Geometry: final body of the model. Coordinates: model frame, mm. Round coordinates to 2 decimals unless told otherwise and drop trailing zeros. Write each loop counter-clockwise with the first axis right and the second up, starting at its lowest first coordinate (ties: lowest second). Pieces come first, ordered by that corner, then holes. Notation, with made-up numbers: (-40, -18.5) -> (5, -18.5) arc R31 cw to (5, 19.5) -> close; hole circle Ø2 at (52, 88). An arc over 180 degrees is marked (long way). Use one line per item in the form item = value. Start each with the question number.
1. Pin query (flat end, axial travel): pin 1 Ø2 at (x, y) = (281.5, 8) entering from -Z; pin 2 Ø2 at (x, z) = (67.5, 15.5) entering from -Y; pin 3 Ø10 at (x, y) = (467.5, 28.5) entering from -Z. Return the tip coordinate at first contact, or that it passes through.
2. Cut plane B-B, the plane z = -9.5. Return the cut outline in (x, y), plus the area to 3 significant figures.
3. Line query: L1, parallel to Y at x = 296, z = -15.5; L2, parallel to Z at x = 364, y = 25; L3, parallel to Y at x = 456, z = 9. Output: solid intervals per line, ascending.
4. Cut plane C-C, the plane y = 27. Return the cut outline in (x, z).
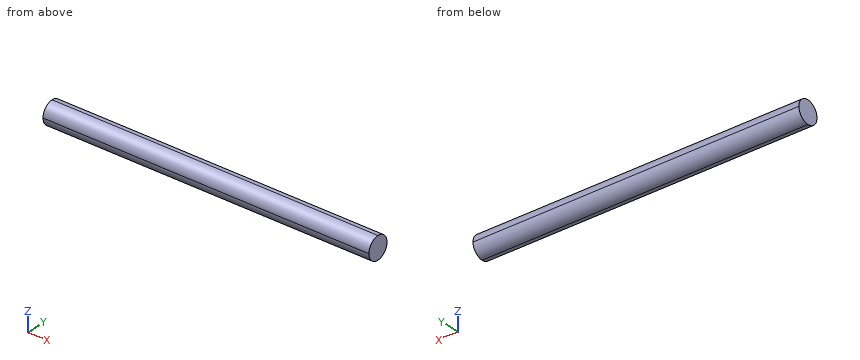
Autodesk Inventor part; units mm, degrees
ref_plane "YZ Plane" through (0, 0, 0) normal (1, 0, 0) x (0, 1, 0)
sketch "1.90 Caprail" plane through (0, 0, 0) normal (0, 0, 1) x (1, 0, 0)
  line L0 (-57.7384, 25.6152) -> (-57.7384, 36.7912) construction
  arc A0 (-65.9934, 36.7912) -> (-67.5174, 35.2672) centre (-65.9934, 35.2672) ccw
  arc A1 (-47.9594, 35.2672) -> (-49.4834, 36.7912) centre (-49.4834, 35.2672) ccw
  arc A2 (-69.8345, 6.4876) -> (-69.016, 6.9384) centre (-69.5494, 6.9384) ccw
  line L1 (-69.016, 6.9384) -> (-69.016, 35.2672)
  arc A3 (-65.9934, 38.2898) -> (-69.016, 35.2672) centre (-65.9934, 35.2672) ccw
  line L2 (-65.9934, 38.2898) -> (-49.4834, 38.2898)
  arc A4 (-46.4608, 35.2672) -> (-49.4834, 38.2898) centre (-49.4834, 35.2672) ccw
  line L3 (-46.4608, 35.2672) -> (-46.4608, 6.9384)
  arc A5 (-46.4608, 6.9384) -> (-45.6423, 6.4876) centre (-45.9274, 6.9384) ccw
  arc A6 (-45.6423, 6.4876) -> (-69.8345, 6.4876) centre (-57.7384, 25.6152) ccw
  line L4 (-47.9594, 6.9384) -> (-47.9594, 35.2672)
  line L5 (-49.4834, 36.7912) -> (-65.9934, 36.7912)
  line L6 (-67.5174, 35.2672) -> (-67.5174, 6.9384)
  arc A7 (-70.5058, 5.1455) -> (-67.5174, 6.9384) centre (-69.5494, 6.9384) ccw
  arc A8 (-47.9594, 6.9384) -> (-44.9711, 5.1455) centre (-45.9274, 6.9384) ccw
  arc A9 (-70.5083, 5.1411) -> (-44.9685, 5.1411) centre (-57.7384, 25.6152) ccw
  circle A10 centre (-57.7384, 25.6152) radius 24.13 construction
  arc A11 (-70.5058, 5.1455) -> (-70.5083, 5.1411) centre (-70.507, 5.1433) ccw
  arc A12 (-44.9685, 5.1411) -> (-44.9711, 5.1455) centre (-44.9699, 5.1433) ccw
  point P0 (-47.9594, 36.7912)
  point P1 (-67.5174, 36.7912)
  dimension "d0" = 48.26
  dimension "d1" = 19.558
  dimension "d2" = 2.032
  dimension "d3" = 11.176
  dimension "d4" = 1.524
  dimension "d5" = 1.4986
  dimension "d6" = 0.0025
sketch "1.66 Caprail" plane through (0, 0, 0) normal (0, 0, 1) x (1, 0, 0)
  arc A0 (55.7245, -3.4499) -> (81.6283, -3.4499) centre (68.6764, 13.1843) ccw
  arc A1 (55.7275, -3.4458) -> (58.8974, -1.7623) centre (56.8654, -1.7623) ccw
  arc A2 (78.4554, -1.7623) -> (81.6253, -3.4458) centre (80.4874, -1.7623) ccw
  line L0 (58.8974, -1.7623) -> (58.8974, 20.8043)
  line L1 (60.4214, 22.3283) -> (76.9314, 22.3283)
  line L2 (78.4554, 20.8043) -> (78.4554, -1.7623)
  line L3 (68.6764, 22.3283) -> (68.6764, 13.1843) construction
  arc A3 (60.4214, 22.3283) -> (58.8974, 20.8043) centre (60.4214, 20.8043) ccw
  arc A4 (78.4554, 20.8043) -> (76.9314, 22.3283) centre (76.9314, 20.8043) ccw
  arc A5 (79.954, -1.7623) -> (80.8181, -2.1808) centre (80.4874, -1.7623) ccw
  line L4 (79.954, -1.7623) -> (79.954, 20.8043)
  arc A6 (79.954, 20.8043) -> (76.9314, 23.8269) centre (76.9314, 20.8043) ccw
  line L5 (76.9314, 23.8269) -> (60.4214, 23.8269)
  arc A7 (60.4214, 23.8269) -> (57.3988, 20.8043) centre (60.4214, 20.8043) ccw
  line L6 (57.3988, 20.8043) -> (57.3988, -1.7623)
  arc A8 (56.5347, -2.1808) -> (57.3988, -1.7623) centre (56.8654, -1.7623) ccw
  arc A9 (80.8181, -2.1808) -> (56.5347, -2.1808) centre (68.6764, 13.1843) ccw
  circle A10 centre (68.6764, 13.1843) radius 21.082 construction
  arc A11 (55.7275, -3.4458) -> (55.7245, -3.4499) centre (55.7261, -3.4479) ccw
  arc A12 (81.6283, -3.4499) -> (81.6253, -3.4458) centre (81.6268, -3.4479) ccw
  point P0 (58.8974, 22.3283)
  point P1 (78.4554, 22.3283)
  dimension "d7" = 42.164
  dimension "d8" = 19.558
  dimension "d9" = 9.144
  dimension "d10" = 2.032
  dimension "d11" = 1.524
  dimension "d12" = 1.4986
  dimension "d13" = 0.0025
sketch "1.50 Caprail" plane through (0, 0, 0) normal (0, 0, 1) x (1, 0, 0)
  arc A0 (154.6368, -0.6357) -> (180.8596, -0.6357) centre (167.7482, 13.1843) ccw
  arc A1 (154.6402, -0.6319) -> (157.9692, 0.9323) centre (155.9372, 0.9323) ccw
  arc A2 (177.5272, 0.9323) -> (180.8562, -0.6319) centre (179.5592, 0.9323) ccw
  circle A3 centre (167.7482, 13.1843) radius 19.05 construction
  arc A4 (179.0258, 0.9323) -> (179.9294, 0.5483) centre (179.5592, 0.9323) ccw
  line L0 (179.0258, 0.9323) -> (179.0258, 23.0903)
  arc A5 (179.0258, 23.0903) -> (176.0032, 26.1129) centre (176.0032, 23.0903) ccw
  line L1 (176.0032, 26.1129) -> (159.4932, 26.1129)
  arc A6 (159.4932, 26.1129) -> (156.4706, 23.0903) centre (159.4932, 23.0903) ccw
  line L2 (156.4706, 23.0903) -> (156.4706, 0.9323)
  arc A7 (155.567, 0.5483) -> (156.4706, 0.9323) centre (155.9372, 0.9323) ccw
  arc A8 (179.9294, 0.5483) -> (155.567, 0.5483) centre (167.7482, 13.1843) ccw
  line L3 (157.9692, 0.9323) -> (157.9692, 23.0903)
  line L4 (159.4932, 24.6143) -> (176.0032, 24.6143)
  line L5 (177.5272, 23.0903) -> (177.5272, 0.9323)
  arc A9 (159.4932, 24.6143) -> (157.9692, 23.0903) centre (159.4932, 23.0903) ccw
  arc A10 (177.5272, 23.0903) -> (176.0032, 24.6143) centre (176.0032, 23.0903) ccw
  line L6 (167.7482, 24.6143) -> (167.7482, 13.1843) construction
  arc A11 (154.6402, -0.6319) -> (154.6368, -0.6357) centre (154.6385, -0.6339) ccw
  arc A12 (180.8596, -0.6357) -> (180.8562, -0.6319) centre (180.8578, -0.6339) ccw
  point P0 (157.9692, 24.6143)
  point P1 (177.5272, 24.6143)
  dimension "d14" = 38.1
  dimension "d15" = 19.558
  dimension "d16" = 2.032
  dimension "d17" = 1.524
  dimension "d18" = 11.43
  dimension "d19" = 1.4986
  dimension "d20" = 0.0025
sketch "1.90 Caprail Outside Edge" plane through (0, 0, 0) normal (0, 0, 1) x (1, 0, 0)
  arc A0 (8.6191, 38.6174) -> (-17.175, 38.6174) centre (-4.278, 59.0116) ccw
  line L0 (5.501, 40.3348) -> (5.501, 68.5975)
  line L1 (3.977, 70.1215) -> (-12.533, 70.1215)
  line L2 (-14.057, 68.5975) -> (-14.057, 40.3348)
  line L3 (-4.278, 59.0116) -> (-4.278, 70.1215) construction
  arc A1 (-17.175, 38.6174) -> (-14.057, 40.3348) centre (-16.089, 40.3348) ccw
  arc A2 (5.501, 40.3348) -> (8.6191, 38.6174) centre (7.533, 40.3348) ccw
  arc A3 (-12.533, 70.1215) -> (-14.057, 68.5975) centre (-12.533, 68.5975) ccw
  arc A4 (5.501, 68.5975) -> (3.977, 70.1215) centre (3.977, 68.5975) ccw
  point P0 (5.501, 70.1215)
  point P1 (-14.057, 70.1215)
  point P2 (-14.057, 36.9519)
  point P3 (5.501, 36.9519)
  dimension "d21" = 13.02
  dimension "d22" = 19.558
  dimension "d23" = 24.13
  dimension "d24" = 2.032
  dimension "d25" = 1.524
sketch "1.66 Caprail Outside Edge" plane through (0, 0, 0) normal (0, 0, 1) x (1, 0, 0)
  arc A0 (-64.2087, 6.8983) -> (-90.3503, 6.8983) centre (-77.2795, 23.4393) ccw
  line L0 (-67.5005, 8.4926) -> (-67.5005, 30.9932)
  line L1 (-69.0245, 32.5172) -> (-85.5345, 32.5172)
  line L2 (-87.0585, 30.9932) -> (-87.0585, 8.4926)
  line L3 (-77.2795, 23.4393) -> (-77.2795, 32.5172) construction
  arc A1 (-90.3503, 6.8983) -> (-87.0585, 8.4926) centre (-89.0905, 8.4926) ccw
  arc A2 (-67.5005, 8.4926) -> (-64.2087, 6.8983) centre (-65.4685, 8.4926) ccw
  arc A3 (-85.5345, 32.5172) -> (-87.0585, 30.9932) centre (-85.5345, 30.9932) ccw
  arc A4 (-67.5005, 30.9932) -> (-69.0245, 32.5172) centre (-69.0245, 30.9932) ccw
  point P0 (-67.5005, 32.5172)
  point P1 (-87.0585, 32.5172)
  point P2 (-87.0585, 4.7625)
  point P3 (-67.5005, 4.7625)
  dimension "d26" = 12.004
  dimension "d27" = 19.558
  dimension "d28" = 21.082
  dimension "d29" = 2.032
  dimension "d30" = 1.524
sketch "1.50 Caprail Outside Edge" plane through (0, 0, 0) normal (0, 0, 1) x (1, 0, 0)
  arc A0 (-129.2922, 11.7711) -> (-155.7348, 11.7711) centre (-142.5135, 25.486) ccw
  line L0 (-132.7345, 13.234) -> (-132.7345, 35.4784)
  line L1 (-134.2585, 37.0024) -> (-150.7685, 37.0024)
  line L2 (-152.2925, 35.4784) -> (-152.2925, 13.234)
  line L3 (-142.5135, 25.486) -> (-142.5135, 37.0024) construction
  arc A1 (-155.7348, 11.7711) -> (-152.2925, 13.234) centre (-154.3245, 13.234) ccw
  arc A2 (-132.7345, 13.234) -> (-129.2922, 11.7711) centre (-130.7025, 13.234) ccw
  arc A3 (-150.7685, 37.0024) -> (-152.2925, 35.4784) centre (-150.7685, 35.4784) ccw
  arc A4 (-132.7345, 35.4784) -> (-134.2585, 37.0024) centre (-134.2585, 35.4784) ccw
  point P0 (-132.7345, 37.0024)
  point P1 (-152.2925, 37.0024)
  point P2 (-152.2925, 9.1375)
  point P3 (-132.7345, 9.1375)
  dimension "d31" = 7.5336
  dimension "d32" = 19.558
  dimension "d33" = 19.05
  dimension "d34" = 2.032
  dimension "d35" = 1.524
sketch "Sketch1" plane through (0, 0, 0) normal (0, 0, 1) x (1, 0, 0)
  line L0 (0, 0) -> (609.6, 0)
  line L1 (609.6, 0) -> (609.6, 42.164)
  line L2 (609.6, 42.164) -> (0, 42.164)
  line L3 (0, 42.164) -> (0, 0)
  dimension "d37" = 42.164
  dimension "d38" = 609.6
extrude "Extrusion1" add sketch "Sketch1" along normal mid plane 42.164
fillet "Fillet1" radius 21.082 4 edges at (304.8, 42.164, -21.082) (304.8, 42.164, 21.082) (304.8, 0, -21.082) (304.8, 0, 21.082)
equation "\"d37\" = PipeOD"
equation "\"d39\" = PipeOD"
equation "\"d41\" = 0.5 * PipeOD"
equation "\"PipeOD\" = 42.164"
equation "\"PipeWallThickness\" = 3.556"
equation "\"Length\" = 609.6"
properties part number "Update_SetBaseQuantity" material "P792.4"
Outcome:
q1.pin_1 = -17.28
q1.pin_2 = 5.78
q1.pin_3 = -20.94
q2.outline = (0, 2.26) -> (609.6, 2.26) -> (609.6, 39.9) -> (0, 39.9) -> close
q2.area = 22,900 mm^2
q3.L1 = 6.79 to 35.37
q3.L2 = -20.71 to 20.71
q3.L3 = 2.02 to 40.15
q4.outline = (0, -20.23) -> (609.6, -20.23) -> (609.6, 20.23) -> (0, 20.23) -> close
